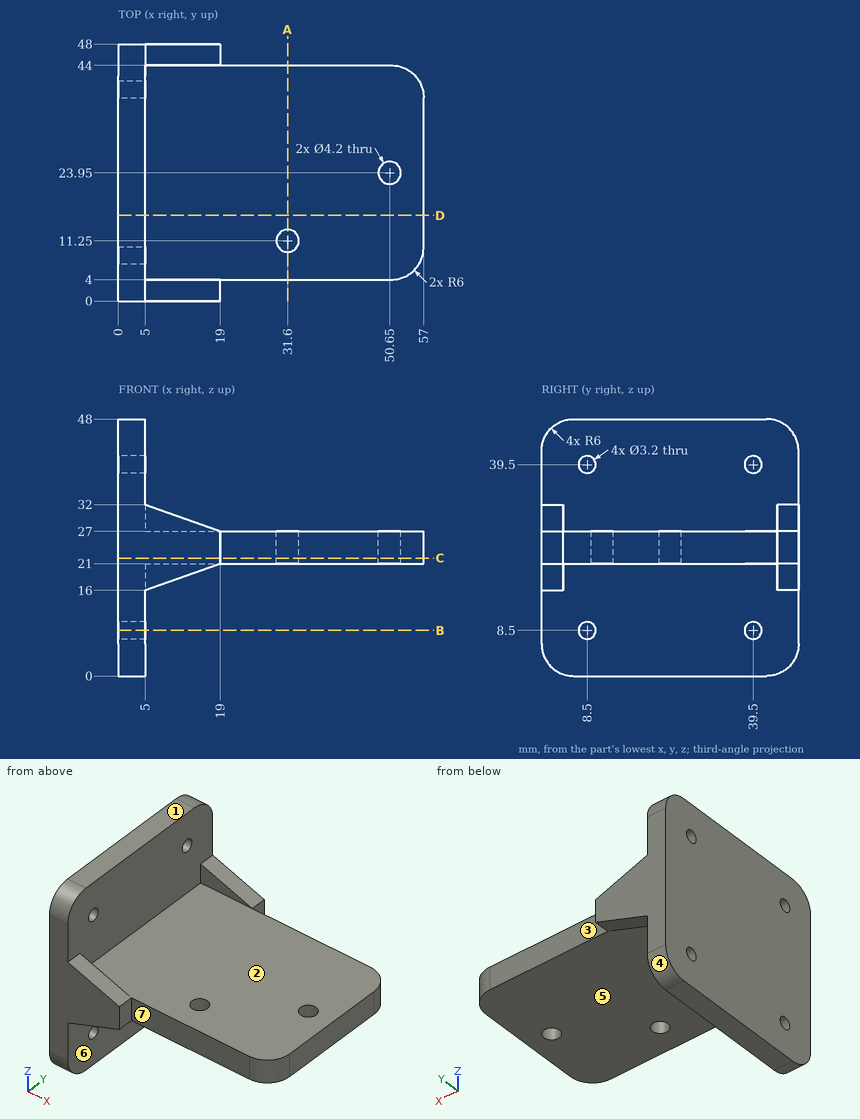
Design review of the part shown in the three views and the two pictorial views. Dimensions are in mm from the part's minimum x, y and z. A direction names the side the tool comes from. Round coordinates to 2 decimals unless told otherwise and drop trailing zeros. Loops run counter-clockwise (first coordinate to the right, second up) from the corner with the lowest first, then second, coordinate; pieces in that order, holes last. Notation, with made-up numbers: (43.25, -5) - (62.25, -5) arc R9 ccw to (62.25, 9) - close; hole circle Ø4 at (-14, -37.75). An arc over 180 degrees is marked (long way). One line per item, written item: value. Start each with the question number.
Item 1: The part is to be moulded in two halves that separate along Y. For the marked faces 4, 5, 6 and 7, say which applies: +Y half, -Y half, draft (parallel to the pull), parting line (faces both ways), or undercut.
Item 2: Take a section at A-A (x = 31.6). Give the boundary of the cut face in (y, z).
Item 3: Take a section at C-C (z = 22). Give the boundary of the cut face in (x, y), plus the area to 3 significant figures.
Item 4: Take a section at B-B (z = 8.5). Give the boundary of the cut face in (x, y).
Item 5: For the marked faces 1, 2 and 3, list the 3-axis set-ups (+Z, -Z, +X, -X, +Y, -Y) from which the entire face can be reached by the end or side of a thin tool; tool diameter is ignored.
Item 6: Take a section at D-D (y = 16). Give the boundary of the cut face in (x, z).
Item 7: Clearance check with flat-ended pins moving along their axes: pin 1 Ø3 at (x, y) = (33.5, 10.5) entering from -Z; pin 2 Ø5 at (x, y) = (46.5, 9) entering from +Z; pin 3 Ø2.5 at (y, z) = (8.5, 8.5) entering from +X; pin 4 Ø2 at (y, z) = (1.5, 23) entering from +X. State where each tip first meets the part, or that it passes through.
Item 8: For L1, parallel to Z at x = 1.65, y = 8.5; L2, parallel to X at y = 11, z = 22; L3, parallel to Y at x = 1, z = 39, list the stretches that pass through material, from the lowest coordinate up.
Answer below:
1. face 4: +Y half
1. face 5: undercut
1. face 6: undercut
1. face 7: -Y half
2. outline: (4, 21) - (9.15, 21) - (9.15, 27) - (4, 27) - close; (13.35, 21) - (44, 21) - (44, 27) - (13.35, 27) - close
3. outline: (0, 0) - (19, 0) - (19, 4) - (51, 4) arc R6 ccw to (57, 10) - (57, 38) arc R6 ccw to (51, 44) - (19, 44) - (19, 48) - (0, 48) - close; hole circle Ø4.2 at (31.6, 11.25); hole circle Ø4.2 at (50.65, 23.95)
3. area: 2,390 mm2
4. outline: (0, 0) - (5, 0) - (5, 6.9) - (0, 6.9) - close; (0, 10.1) - (5, 10.1) - (5, 37.9) - (0, 37.9) - close; (0, 41.1) - (5, 41.1) - (5, 48) - (0, 48) - close
5. face 1: +Z, +X, -X, +Y, -Y
5. face 2: +Z, +X
5. face 3: +Z, -Z, +X, +Y
6. outline: (0, 0) - (5, 0) - (5, 21) - (57, 21) - (57, 27) - (5, 27) - (5, 48) - (0, 48) - close
7. pin 1: stops at z = 21
7. pin 2: stops at z = 27
7. pin 3: passes through
7. pin 4: stops at x = 19
8. L1: z = 0 to 6.9, 10.1 to 37.9, 41.1 to 48
8. L2: x = 0 to 29.51, 33.69 to 57
8. L3: y = 0 to 6.98, 10.02 to 37.98, 41.02 to 48
